Source: CAD feature listing. Evaluate the final solid. Frame: model axes, mm. A direction names the side the tool comes from. Give positions to 0.01 mm unless a question says otherwise; leave off trailing zeros. Order: outer loops, then holes, each group sorted by start corner. A loop starts at its lowest first (then second) coordinate and runs counter-clockwise, first axis right, second up. Notation, with made-up numbers: M 84.25,44 L 119.25,44 A23 cw 119.25,73 Z; hole C -21,14.5 d4. An arc over 180 degrees is marked long. Answer in a Markdown table with one row per item. Add a question column.
(1) Section query D-D, the plane x = 5.25. Return loops of the section in (y, z) (3 decimals), plus the area to 3 significant figures.
(2) Section query B-B, the plane y = 2. Return loops of the section in (x, z) (3 decimals), plus the area to 3 significant figures.
(3) Material intervals for line 1 along X through (y, z) = (0, 2.95) (1 decimal); line 2 along X through (y, z) = (0, 7.6) (1 decimal), sorted ascending.
(4) Set-up query: faces 4 (the face through (0.748, -0.976, 1.932)), 5 (the face through (0.086, 0.078, 6.944)), 6 (the face through (2.04, 0.16, 6.58)). Return all of +Z, -Z, +X, -X, +Y, -Y with unobstructed straight access to the full face (end or side cutting, diameter ignored); none if empty.
(5) Pin query (flat end, axial travel): P1, Ø1.5, axis at x = 3, y = 2, coming from the -Z side; P2, Ø1.5, axis at y = -2.5, z = 5.5, coming from the -X side; P3, Ø1.5, axis at x = 3.26, y = 0, coming from the +Z side; P4, Ø1.5, axis at x = 0, y = 0, coming from the -Z side. Return the tip coordinate at first contact, or that it passes through.
(6) Mould query, pull axis X, two halves, no side actions, for faces 1 (the face through (-2.8, 1.5, 2)), 2 (the face through (3.05, 0.05, 4.09)), 3 (the face through (4, 0, 3.175)). Classes: pulls with the +X half, pulls with the -X half, needs draft (parallel to the pull), parting line crosses it, or undercut.
Autodesk Inventor part; units mm, degrees
ref_plane "YZ Plane" through (0, 0, 0) normal (1, 0, 0) x (0, 1, 0)
ref_plane "XZ Plane" through (0, 0, 0) normal (0, 1, 0) x (-1, 0, 0)
ref_plane "XY Plane" through (0, 0, 0) normal (0, 0, 1) x (1, 0, 0)
sketch "Sketch2" plane through (0, 0, 0) normal (0, 0, 1) x (1, 0, 0)
  arc A0 (3.26, -3.175) -> (3.26, 3.175) centre (3.26, 0) ccw
  arc A1 (0, 3.175) -> (0, -3.175) centre (0, 0) ccw
  line L0 (0, 3.175) -> (3.26, 3.175)
  line L1 (0, -3.175) -> (3.26, -3.175)
  dimension "d14" = 6.35
  dimension "d15" = 6.35
  dimension "d16" = 0
  dimension "d17" = 0
  dimension "d18" = 3.26
  dimension "d19" = 0
extrude "Extrusion2" add sketch "Sketch2" along normal blind 8.509
sketch "Sketch3" plane through (0, 0, 8.509) normal (0, 0, 1) x (1, 0, 0)
  point P0 (0, 0)
  point P1 (3.26, 0)
  dimension "d22" = 3.26
  dimension "d23" = 0
hole "Hole1" at (3.26, 0, 8.509) direction (0, 0, -1) diameter 2.459 depth 3.81 tip angle 118
sketch "Sketch4" plane through (0, 0, 0) normal (0, 0, -1) x (-1, 0, 0)
  point P0 (0, 0)
hole "Hole2" at (0, 0, 0) direction (0, 0, 1) diameter 2.459 depth 3.81 tip angle 118
sketch "Sketch5" plane through (0, 0, 0) normal (0, 0, -1) x (-1, 0, 0)
  arc A0 (-3.26, 3.175) -> (-3.26, -3.175) centre (-3.26, 0) ccw
  arc A1 (0, 3.175) -> (0, -3.175) centre (0, 0) ccw
  line L0 (0, 3.175) -> (-3.26, 3.175)
  arc A2 (0, -3.175) -> (0, 3.175) centre (0, 0) ccw
  line L1 (0, -3.175) -> (-3.26, -3.175)
  dimension "d42" = 3.26
extrude "Extrusion3" cut sketch "Sketch5" against normal blind 3.175 from surface at 0 contours L0 A1 L1 A0
sketch "Sketch6" plane through (0, 0, 8.509) normal (0, 0, 1) x (1, 0, 0)
  arc A0 (3.26, 3.175) -> (3.2432, -3.175) centre (3.26, 0) ccw
  line L0 (3.26, 3.175) -> (0, 3.175)
  line L1 (0, -3.175) -> (3.26, -3.175)
  line L2 (3.2432, -3.175) -> (0, -3.175)
  arc A1 (0, 3.175) -> (0, -3.175) centre (0, 0) ccw
  point P0 (3.268, -3.175)
  dimension "d43" = 3.26
extrude "Extrusion4" cut sketch "Sketch6" against normal blind 3.175
properties part number "PC104_EM-113 standoff_3.268" material "Aluminum 6061"
Values follow:
| question | item | result |
|---|---|---|
| 1 | outline | M -2.474,3.175 L 2.474,3.175 L 2.474,8.509 L -2.474,8.509 Z |
| 1 | area | 26.4 mm² |
| 2 | outline | M -2.466,0 L 2.466,0 L 2.466,3.175 L 5.726,3.175 L 5.726,8.509 L 0.794,8.509 L 0.794,5.334 L -2.466,5.334 Z |
| 2 | area | 49.0 mm² |
| 3 | line 1 | x = -3.2 to -1.2, 1.2 to 3.2 |
| 3 | line 2 | x = 0.1 to 2, 4.5 to 6.4 |
| 4 | face 4 | -Z |
| 4 | face 5 | +Z, -X |
| 4 | face 6 | +Z |
| 5 | P1 | stops at z = 0 |
| 5 | P2 | stops at x = -2.64 |
| 5 | P3 | stops at z = 4.41 |
| 5 | P4 | stops at z = 4.1 |
| 6 | face 1 | parting line crosses it |
| 6 | face 2 | undercut |
| 6 | face 3 | needs draft |
